The model under review builds one solid part; all positions refer to its coordinate system, in mm. Face numbers are marked on the shaded views. A direction names the side the tool comes from. Coordinates: 2 decimals unless noted, no trailing zeros. Write each loop counter-clockwise with the first axis right and the second up, starting at its lowest first coordinate (ties: lowest second). Pieces come first, ordered by that corner, then holes. Notation, with made-up numbers: (87, -34.75) - (115, -34.75) arc R3 ccw to (115, -29.75) - close; hole circle Ø11 at (28, 77.5). An arc over 180 degrees is marked (long way). Answer as CSV lines item,"result". Start each with the question number.
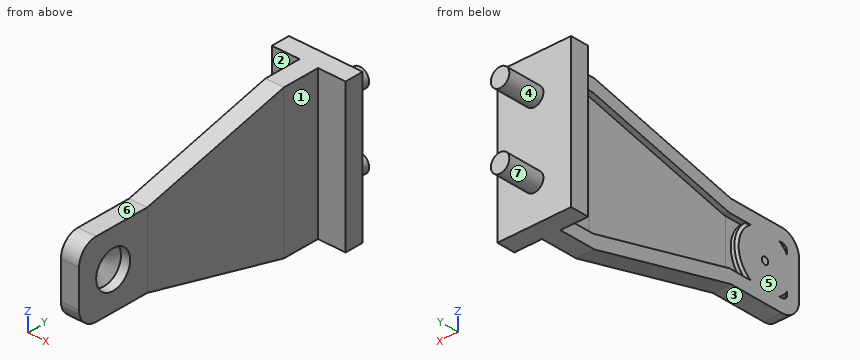
```python
from build123d import *

# Parameters (mm, degrees)
F0_W         = 25.4
F0_H         = 50.8
F1_DEPTH     = 6.35
F2_W         = 6.35
F2_H         = 50.8
F3_DEPTH     = 12.7
F3_FACE_W    = 6.35
F3_FACE_H    = 50.8
F5_W         = 6.2655590393
F5_H         = 25.4
F7_DEPTH     = 25.4
F8_T1_DEPTH  = 38.0155590393
F10_D        = 12.7
F10_DEPTH    = 3.175
F10_TIP      = 3.8154649308
F11_T        = 4.445
F11_T3_DEPTH = 59.69
F11_T5_DEPTH = 15.1555590393
F11_T7_DEPTH = 34.29
F12_R        = 3.175
F13_DEPTH    = 12.7


# Not quite as in the source:
# - a fillet or chamfer that OpenCascade refuses, or shapes differently, is made with other operations: its cross-section is extruded or revolved along the edge and cut away or added
# - a shell that OpenCascade refuses in one call is made with other operations: the cavity is built on its own and cut out


with BuildPart() as f1:
    # F0 (on Front) → F1 (new body)
    with BuildSketch(Plane.XZ):
        with Locations((-6.5905367956, 12.3420813114)):
            Rectangle(F0_W, F0_H)
    extrude(amount=F1_DEPTH)

    # F2 (on face) → F3 (join)
    with BuildSketch(Plane.XZ.offset(6.35)):
        with Locations((-6.5905367956, 12.3420813114)):
            Rectangle(F2_W, F2_H)
    extrude(amount=F3_DEPTH)

    # F3_face (on face) → F6 section 0
    with BuildSketch(Plane(origin=(-6.5905367956, -19.05, 12.3420813114), x_dir=(1, 0, 0), z_dir=(0, -1, 0))):
        Rectangle(F3_FACE_W, F3_FACE_H)
    # F5 (on offset) → F6 section 1
    with BuildSketch(Plane.XZ.offset(69.85)):
        with Locations((-6.6327572759, 12.3420813114)):
            Rectangle(F5_W, F5_H)
    loft()

    # F7 (add): a face of the model
    f7_faces = [f1.faces().sort_by_distance(p)[0] for p in [
        (-6.6327572759, -69.85, 12.3420813114),
    ]]
    extrude(f7_faces, amount=F7_DEPTH)

    # F8: fillet of radius 6.35 on 4 edges, made by hand

    # F8_s2 → F8_t1 (cut)
    with BuildSketch(Plane.YZ.offset(-25.6405367956)):
        with BuildLine():
            ThreePointArc((-88.9, 25.0420813114), (-93.3901280605, 23.1822093719), (-95.25, 18.6920813114))
            Line((-95.25, 18.6920813114), (-95.25, 25.0420813114))
            Line((-95.25, 25.0420813114), (-88.9, 25.0420813114))
        make_face()
        with BuildLine():
            ThreePointArc((-88.9, -0.3579186886), (-93.3901280605, 1.5019532508), (-95.25, 5.9920813114))
            Line((-95.25, 5.9920813114), (-95.25, -0.3579186886))
            Line((-95.25, -0.3579186886), (-88.9, -0.3579186886))
        make_face()
    extrude(amount=F8_T1_DEPTH, mode=Mode.SUBTRACT)

    # F10
    with Locations(Plane.YZ.offset(-3.4999777563)):
        with Locations((-82.55, 12.3420813114)):
            Hole(F10_D / 2, depth=F10_DEPTH)
            with Locations((0, 0, -(F10_DEPTH + F10_TIP / 2))):  # 118° drill point
                Cone(0, F10_D / 2, F10_TIP, mode=Mode.SUBTRACT)

    # F11: shell of thickness 4.445, made by hand


with BuildPart() as f11_core1:
    # F11_t2: copy of F1
    add(f1.part)

    # the walls: a layer under each face that stays
    f11_faces = [f11_core1.faces().sort_by_distance(p)[0] for p in [
        (-19.2905367956, -3.175, 12.3420813114),
        (-6.5905367956, -9.525, 37.7420813114),
        (-6.5905367956, -9.525, -13.0579186886),
        (-6.5905367956, 0, 12.3420813114),
        (-14.5280367956, -6.35, 12.3420813114),
        (6.1094632044, -3.175, 12.3420813114),
        (1.3469632044, -6.35, 12.3420813114),
        (-3.4155367956, -12.7, 12.3420813114),
        (-6.6116470357, -44.45, 31.3920813114),
        (-6.6116470357, -44.45, -6.7079186886),
        (-3.4577572759, -44.45, 12.3420813114),
        (-6.6327572759, -79.375, 25.0420813114),
        (-6.6327572759, -79.375, -0.3579186886),
        (-6.6327572759, -93.3901280605, 23.1822093719),
        (-6.6327572759, -93.3901280606, 1.5019532508),
        (-6.6327572759, -95.25, 12.3420813114),
        (-8.2202572759, -86.328223001, 12.3420813114),
        (-3.4999777563, -91.0166666667, 3.8754146447),
        (-5.0874777563, -88.9, 12.3420813114),
    ]]
    thicken(f11_faces, amount=-F11_T, mode=Mode.SUBTRACT)

    # F11_s4 → F11_t3 (cut)
    with BuildSketch(Plane.XY.offset(-17.5029186886)):
        Polygon((-3.3710867956, -6.39445), (-3.4155367956, -1.905), (-7.8605367956, -1.905), (-7.8605367956, -6.35), align=None)
    extrude(amount=F11_T3_DEPTH, mode=Mode.SUBTRACT)

    # F11_s6 → F11_t5 (cut)
    with BuildSketch(Plane.YZ.offset(-14.2105367956)):
        Polygon((-69.8607807085, 25.1296541455), (-68.7719291467, 20.7297978982), (-69.3027954941, 20.5970813114), (-69.85, 20.5970813114), align=None)
        Polygon((-69.8607807085, -0.4454915228), (-68.7719291467, 3.9543647245), (-69.3027954941, 4.0870813114), (-69.85, 4.0870813114), align=None)
    extrude(amount=F11_T5_DEPTH, mode=Mode.SUBTRACT)

    # F11_s8 → F11_t7 (cut)
    with BuildSketch(Plane.XY.offset(-4.8029186886)):
        Polygon((-3.4110778177, -69.8500738857), (-7.9449716156, -69.8426114261), (-7.9449777563, -69.8463057105), (-7.9449777563, -69.85), align=None)
    extrude(amount=F11_T7_DEPTH, mode=Mode.SUBTRACT)

    # F11_s9 → F11_t10 (revolve, cut)
    with BuildSketch(Plane.XY.offset(12.3420813114)):
        Polygon((-6.6368766698, -76.2673434424), (-10.4850864079, -73.910655757), (-9.1898377553, -71.755), (-6.6749777563, -71.755), align=None)
    revolve(axis=Axis((-6.6749777563, -82.55, 12.3420813114), (1, 0, 0)), mode=Mode.SUBTRACT)


with BuildPart() as f1_1:
    add(f1.part)

    # what is left inside the walls is the cavity
    f11_cavity = [f11_core1.part.solids().sort_by_distance(p)[0] for p in [
        (-9.721087, -28.696773, 12.342081),
        (-9.611738, -89.747742, 5.14434),
        (-9.611738, -89.747742, 19.539823),
    ]]
    add(f11_cavity, mode=Mode.SUBTRACT)

    # F12 (on face) → F13 (join)
    with BuildSketch(Plane(origin=(0, 0, 0), x_dir=(-1, 0, 0), z_dir=(0, 1, 0))):
        with Locations((6.5905367956, 25.0420813114)):
            Circle(F12_R)
        with Locations((6.5905367956, -0.3579186886)):
            Circle(F12_R)
    extrude(amount=F13_DEPTH)


solid = f1_1.part
```
(1) The part is to be moulded in two halves that separate along Z. For the marked faces 4, 5, 6 and 7, say which applies: released by +Z, released by -Z, zero draft, split by the parting line, or undercut.
(2) For pin 1 (10 mm diameter, centred on x = -11, y = -65.5, fed in from +Z); pin 2 (14 mm diameter, centred on y = -11, z = 14, fed in from +X); pin 3 (4 mm diameter, centred on x = -15.5, z = 6.5, fed in from +Y); pin 4 (7 mm diameter, centred on x = -5.5, y = -75, fed in from -Z), all flat-tipped, find the tip position at first contact; note any pin that passes through.
(3) Add section C-C on x = -16.5. Give the boundary of the cut face in (y, z), then the cut area to 3 significant figures.
(4) Add section B-B on y = -8. Give the boundary of the cut face in (x, z).
(5) For the marked faces 1, 2 and 3, list the 3-axis set-ups (+Z, -Z, +X, -X, +Y, -Y) from which the entire face can be reached by the end or side of a thin tool; tool diameter is ignored.
(6) Wall thickness on line 1 (Z direction, x = -4.65, y = -82.55); line 2 (Y direction, x = -15.75, z = -2); line 3 (X direction, y = -32, z = 32): over which ranges is each line inside the solid? List them lowest first.
(7) Add section A-A on y = -82.55. Give the boundary of the cut face in (x, z).
Reported:
1,face 4,"undercut"
1,face 5,"zero draft"
1,face 6,"released by +Z"
1,face 7,"undercut"
2,pin 1,"z = 27.34"
2,pin 2,"x = 6.11"
2,pin 3,"y = 0"
2,pin 4,"z = -0.36"
3,outline,"(-6.35, -13.06) - (0, -13.06) - (0, 37.74) - (-6.35, 37.74) - close"
3,area,"323 mm²"
4,outline,"(-9.77, -13.06) - (-3.42, -13.06) - (-3.42, 37.74) - (-9.77, 37.74) - (-9.77, 33.3) - (-7.86, 33.3) - (-7.86, -8.61) - (-9.77, -8.61) - close"
5,face 1,"+Z, -Z, +X, -Y"
5,face 2,"+Z, -Z, -X, -Y"
5,face 3,"-Z, +X, -X, -Y"
6,line 1,"-0.36 to 5.99, 18.69 to 25.04"
6,line 2,"-6.35 to 0"
6,line 3,"-9.77 to -3.44"
7,outline,"(-9.77, -0.36) - (-3.5, -0.36) - (-3.5, 5.99) - (-6.67, 5.99) - (-9.77, 11.14) - close; (-9.77, 13.55) - (-6.67, 18.69) - (-3.5, 18.69) - (-3.5, 25.04) - (-9.77, 25.04) - close"
